```python
from build123d import *

# Parameters (mm, degrees)
ESBO_O1_W                = 49
ESBO_O1_H                = 35
RESSALTO_EXTRUS_O1_DEPTH = 3
ESBO_O2_R                = 1.35
CORTE_EXTRUS_O1_DEPTH    = 31.257230541
ESBO_O3_W                = 49
ESBO_O3_H                = 3
RESSALTO_EXTRUS_O3_DEPTH = 8
ESBO_O4_R                = 1.35
CORTE_EXTRUS_O2_DEPTH    = 44.465503563
FILETE1_R                = 2
FILETE2_R                = 2


with BuildPart() as part:
    # Esboço1 → Ressalto-extrusão1 (new body)
    with BuildSketch(Plane.XY):
        Rectangle(ESBO_O1_W, ESBO_O1_H)
    extrude(amount=RESSALTO_EXTRUS_O1_DEPTH)

    # Esboço2 → Corte-extrusão1 (cut, through all)
    with BuildSketch(Plane(origin=(0, 0, 0), x_dir=(-1, 0, 0), z_dir=(0, 0, -1))):
        with Locations((-21.9, -14.9)):
            Circle(ESBO_O2_R)
        with Locations((0, -14.9)):
            Circle(ESBO_O2_R)
        with Locations((21.9, -14.9)):
            Circle(ESBO_O2_R)
    extrude(amount=-CORTE_EXTRUS_O1_DEPTH, mode=Mode.SUBTRACT)

    # Esboço3 → Ressalto-extrusão3 (add)
    with BuildSketch(Plane(origin=(0, 0, 0), x_dir=(-1, 0, 0), z_dir=(0, 0, -1))):
        with Locations((0, 16)):
            Rectangle(ESBO_O3_W, ESBO_O3_H)
    extrude(amount=RESSALTO_EXTRUS_O3_DEPTH)

    # Esboço4 → Corte-extrusão2 (cut, through all)
    with BuildSketch(Plane(origin=(0, 17.5, 0), x_dir=(1, 0, 0), z_dir=(0, 1, 0))):
        with Locations(Location((-21.9, 5.4, 0), (0, 0, 270))):
            Circle(ESBO_O4_R)
        with Locations(Location((0, 5.4, 0), (0, 0, 270))):
            Circle(ESBO_O4_R)
        with Locations(Location((21.9, 5.4, 0), (0, 0, 270))):
            Circle(ESBO_O4_R)
    extrude(amount=-CORTE_EXTRUS_O2_DEPTH, mode=Mode.SUBTRACT)

    # Filete1
    filete1_edges = [part.edges().sort_by_distance(p)[0] for p in [
        (24.5, -17.5, 1.5),
        (-24.5, -17.5, 1.5),
    ]]
    fillet(filete1_edges, radius=FILETE1_R)

    # Filete2
    filete2_edges = [part.edges().sort_by_distance(p)[0] for p in [
        (24.5, 16, -8),
        (-24.5, 16, -8),
    ]]
    fillet(filete2_edges, radius=FILETE2_R)


solid = part.part
```
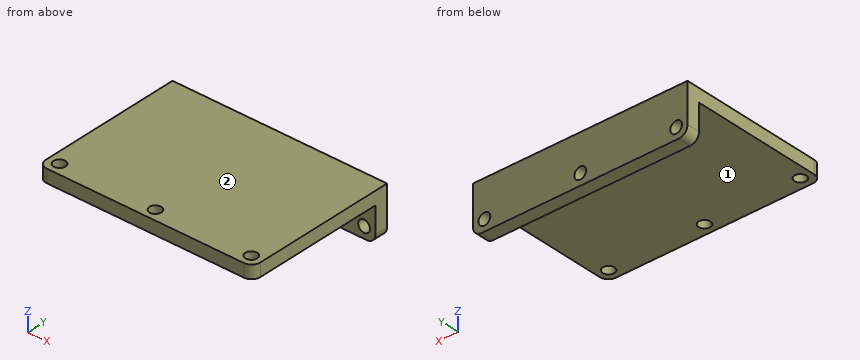
The listing builds one solid part. Answer for the finished solid, in the listing's coordinates (mm). Face numbers are marked on the shaded views. A direction names the side the tool comes from. Round coordinates to 2 decimals unless told otherwise and drop trailing zeros. Loops run counter-clockwise (first coordinate to the right, second up) from the corner with the lowest first, then second, coordinate; pieces in that order, holes last. Notation, with made-up numbers: (28.5, 28) - (78.5, 28) arc R33 cw to (78.5, 57) - close; hole circle Ø7 at (44, 58). An arc over 180 degrees is marked (long way). Return JSON: item names as keys, results as strings. Group by question number.
1. The part is cut by section B-B on x = -21.9. Determine the outline of the cut face in (y, z), then the cut area to 3 significant figures.
2. The part is cut by section A-A on y = -14.9. Determine the outline of the cut face in (x, z).
3. Which of the six approach directions +Z, -Z, +X, -X, +Y, -Y give full straight-line access (tool end or side, diameter ignored) to the marked faces 1 and 2?
4. Each of these flat-tipped pins is pushed along its axis until it touches: P1, Ø2.5, axis at x = 21.9, y = -14.9, coming from the +Z side; P2, Ø3, axis at x = 21.9, z = -5.4, coming from the -Y side; P3, Ø16, axis at x = 6.5, y = -0.5, coming from the -Z side. Where does it stop, or does it pass through?
5. Consider probe 1 along X at (y, z) = (16.05, -5.4); probe 2 along Y at (x, z) = (21.9, 1.9); probe 3 along Z at (x, y) = (-2, 10). Determine where each line is inside the solid, lowest interval first.
6. The part is cut by section C-C on z = -5.4. Determine the outline of the cut face in (x, y), then the cut area to 3 significant figures.
7. The part is cut by section D-D on x = -11. Determine the outline of the cut face in (y, z), then the cut area to 3 significant figures.
Resolved:
{
 "1": {"outline": "(-17.5, 0) - (-16.25, 0) - (-16.25, 3) - (-17.5, 3) - close; (-13.55, 0) - (14.5, 0) - (14.5, -4.05) - (17.5, -4.05) - (17.5, 3) - (-13.55, 3) - close; (14.5, -8) - (17.5, -8) - (17.5, -6.75) - (14.5, -6.75) - close", "area": "113 mm²"},
 "2": {"outline": "(-24.5, 0) - (-23.25, 0) - (-23.25, 3) - (-24.5, 3) - close; (-20.55, 0) - (-1.35, 0) - (-1.35, 3) - (-20.55, 3) - close; (1.35, 0) - (20.55, 0) - (20.55, 3) - (1.35, 3) - close; (23.25, 0) - (24.5, 0) - (24.5, 3) - (23.25, 3) - close"},
 "3": {"face 1": "-Z, +X, -X, -Y", "face 2": "+Z, +X, -X, +Y, -Y"},
 "4": {"P1": "passes through", "P2": "stops at y = 14.5", "P3": "stops at z = 0"},
 "5": {"probe 1": "x = -24.5 to -23.25, -20.55 to -1.35, 1.35 to 20.55, 23.25 to 24.5", "probe 2": "y = -17.5 to -16.25, -13.55 to 17.5", "probe 3": "z = 0 to 3"},
 "6": {"outline": "(-24.5, 14.5) - (-23.25, 14.5) - (-23.25, 17.5) - (-24.5, 17.5) - close; (-20.55, 14.5) - (-1.35, 14.5) - (-1.35, 17.5) - (-20.55, 17.5) - close; (1.35, 14.5) - (20.55, 14.5) - (20.55, 17.5) - (1.35, 17.5) - close; (23.25, 14.5) - (24.5, 14.5) - (24.5, 17.5) - (23.25, 17.5) - close", "area": "123 mm²"},
 "7": {"outline": "(-17.5, 0) - (14.5, 0) - (14.5, -8) - (17.5, -8) - (17.5, 3) - (-17.5, 3) - close", "area": "129 mm²"}
}
